from build123d import *

# Parameters (mm, degrees)
SKETCH3_R          = 1.6
CUT_EXTRUDE1_DEPTH = 11.932634632
CIRPATTERN1_COUNT  = 6


with BuildPart() as part:
    # Sketch1 → Revolve1 (revolve)
    with BuildSketch(Plane(origin=(0, 0, 0), x_dir=(0, 0, -1), z_dir=(1, 0, 0)), mode=Mode.PRIVATE) as revolve1_sk:
        Polygon((0, 0.5), (0, 2.05), (1.8, 2.05), (1.8, 7.5), (2.65, 7.5), (2.65, 1.5), (3, 1.5), (3, 0.5), align=None)
    revolve(revolve1_sk.sketch.rotate(Axis((0, 0, 128.698308515), (0, 0, -1)), 90), axis=Axis((0, 0, 128.698308515), (0, 0, -1)))

    # Sketch3 → Cut-Extrude1 (cut, through all)
    with BuildSketch(Plane(origin=(0, 0, -2.65), x_dir=(-1, 0, 0), z_dir=(0, 0, -1))):
        with Locations((0, 4.3)):
            Circle(SKETCH3_R)
    cut_extrude1 = extrude(amount=-CUT_EXTRUDE1_DEPTH, mode=Mode.SUBTRACT)

    # CirPattern1: Cut-Extrude1 ×6 about axis
    cirpattern1_axis = Axis((0, 0, 0), (0, 0, 1))
    for i in range(1, CIRPATTERN1_COUNT):
        add(cut_extrude1.rotate(cirpattern1_axis, i * 360 / CIRPATTERN1_COUNT), mode=Mode.SUBTRACT)


solid = part.part
Here's how the part is built. I have some questions about the finished solid (model axes, mm). A direction names the side the tool comes from. Give positions to 0.01 mm unless a question says otherwise; leave off trailing zeros. Order: outer loops, then holes, each group sorted by start corner. A loop starts at its lowest first (then second) coordinate and runs counter-clockwise, first axis right, second up. Notation, with made-up numbers: M 26.25,-23 L 66.25,-23 A17 cw 66.25,-18 Z; hole C -4.75,40.25 d7. An arc over 180 degrees is marked long. Answer as a JSON object with one key per item and string values. Group by question number.
1) We'd pull the mould along Y, two halves only. Please class faces 3 (the cylindrical face through (1.43, -0.45, -2.83)), 4 (the cylindrical face through (-3.516, -0.564, -2.231)), 5 (the flat face through (1, 0, -3)): pulls with the +Y half, pulls with the -Y half, needs draft (parallel to the pull), parting line crosses it, or undercut.
2) Suppose I cut it at D-D, the plane z = -1.45. Write out the boundary of the cut face in (x, y), plus the area to 3 significant figures.
3) On a 3-axis mill with a long thin cutter (end or side, diameter ignored), from which of +Z, -Z, +X, -X, +Y, -Y can I reach the whole of each face in a straight line? I mean faces 1 (the cylindrical face through (-0.35, -2.74, -2.23)), 2 (the cylindrical face through (-0.267, -2.033, -0.913)). Say none if no direction works.
4) Suppose I cut it at C-C, the plane x = -2.5. Write out the boundary of the cut face in (y, z), plus the area to 3 significant figures.
5) Please list where these lines run through material, in increasing order: L1, parallel to Y at x = 0, z = -2.3; L2, parallel to Z at x = -5.75, y = 1.75; L3, parallel to Y at x = 4.25, z = -2.05. Write a range as [from, to].
6) Suppose I cut it at A-A, the plane y = 0. Write out the boundary of the cut face in (x, z).
7) Suppose I cut it at B-B, the plane x = 0. Write out the boundary of the cut face in (y, z).
8) I'm going to push flat-ended pins straight in: pin 1 Ø1.9 at (x, y) = (0, -4.3) entering from +Z; pin 2 Ø4.5 at (x, y) = (3.5, -2.5) entering from -Z; pin 3 Ø1 at (y, z) = (1, -1) entering from -X; pin 4 Ø4 at (x, y) = (-3.72, -2.15) entering from +Z. Where does each tip first touch, or does it pass through?
Results found:
{
 "1": {"face 3": "parting line crosses it", "face 4": "undercut", "face 5": "needs draft"},
 "2": {"outline": "C 0,0 d4.1; hole C 0,0 d1", "area": "12.4 mm²"},
 "3": {"face 1": "+Z, -Z", "face 2": "+Z"},
 "4": {"outline": "M -7.07,-2.65 L -3.18,-2.65 L -3.18,-1.8 L -7.07,-1.8 Z; M -1.12,-2.65 L 1.12,-2.65 L 1.12,-1.8 L -1.12,-1.8 Z; M 3.18,-2.65 L 7.07,-2.65 L 7.07,-1.8 L 3.18,-1.8 Z", "area": "8.52 mm²"},
 "5": {"L1": "[-7.5, -5.9], [-2.7, -0.5], [0.5, 2.7], [5.9, 7.5]", "L2": "[-2.65, -1.8]", "L3": "[-6.18, -3.66], [-0.64, 0.64], [3.66, 6.18]"},
 "6": {"outline": "M -7.5,-2.65 L -1.5,-2.65 L -1.5,-3 L -0.5,-3 L -0.5,0 L -2.05,0 L -2.05,-1.8 L -7.5,-1.8 Z; M 0.5,-3 L 1.5,-3 L 1.5,-2.65 L 7.5,-2.65 L 7.5,-1.8 L 2.05,-1.8 L 2.05,0 L 0.5,0 Z"},
 "7": {"outline": "M -7.5,-2.65 L -5.9,-2.65 L -5.9,-1.8 L -7.5,-1.8 Z; M -2.7,-2.65 L -1.5,-2.65 L -1.5,-3 L -0.5,-3 L -0.5,0 L -2.05,0 L -2.05,-1.8 L -2.7,-1.8 Z; M 0.5,-3 L 1.5,-3 L 1.5,-2.65 L 2.7,-2.65 L 2.7,-1.8 L 2.05,-1.8 L 2.05,0 L 0.5,0 Z; M 5.9,-2.65 L 7.5,-2.65 L 7.5,-1.8 L 5.9,-1.8 Z"},
 "8": {"pin 1": "through", "pin 2": "z = -2.65", "pin 3": "x = -1.99", "pin 4": "z = -1.8"}
}
